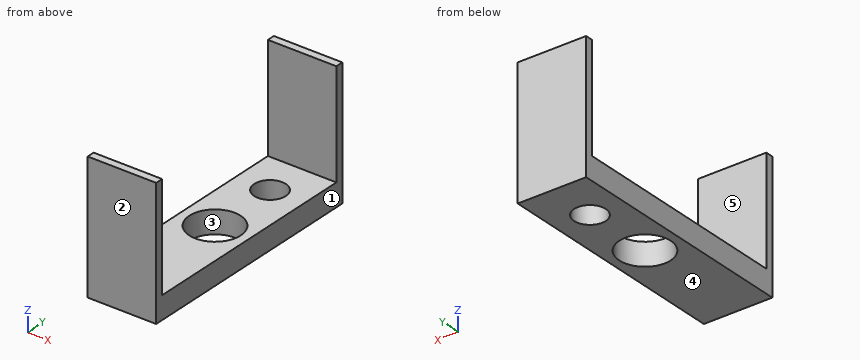
```python
from build123d import *

# Parameters (mm, degrees)
F0_W     = 24
F0_H     = 84.54
F1_DEPTH = 8
F2_W     = 24
F2_H     = 2.7
F3_DEPTH = 37.2
F4_R     = 9
F5_DEPTH = 8.001
F6_R     = 5.524405
F7_DEPTH = 8.001


with BuildPart() as f1:
    # F0 (on Top) → F1 (new body)
    with BuildSketch(Plane.XY):
        Rectangle(F0_W, F0_H)
    extrude(amount=F1_DEPTH)

    # F2 (on face) → F3 (join)
    with BuildSketch(Plane.XY.offset(8)):
        with Locations((0, 40.92)):
            Rectangle(F2_W, F2_H)
        with Locations((0, -40.92)):
            Rectangle(F2_W, F2_H)
    extrude(amount=F3_DEPTH)

    # F4 (on face) → F5 (cut, through all)
    with BuildSketch(Plane.XY.offset(8)):
        Circle(F4_R)
    extrude(amount=-F5_DEPTH, mode=Mode.SUBTRACT)

    # F6 (on face) → F7 (cut, through all)
    with BuildSketch(Plane.XY.offset(8)):
        with Locations((0, 25)):
            Circle(F6_R)
    extrude(amount=-F7_DEPTH, mode=Mode.SUBTRACT)


solid = f1.part
```
Can you work these out from the model? Positions are in its coordinate system, mm. Face numbers are marked on the shaded views. A direction names the side the tool comes from. Coordinates: 2 decimals unless noted, no trailing zeros. Order: outer loops, then holes, each group sorted by start corner. A loop starts at its lowest first (then second) coordinate and runs counter-clockwise, first axis right, second up.
1. If we section it at D-D (x = 7): Please give me the cut outline in (y, z), then the cut area to 3 significant figures.
2. Thinking about a two-plate mould opening in X: for the marked faces 1, 2 and 3, which applies, +X half, -X half, draft (parallel to the pull), parting line (faces both ways), or undercut?
3. If we section it at B-B (x = 0): Please give me the cut outline in (y, z), then the cut area to 3 significant figures.
4. For the marked faces 4 and 5, which set-ups out of +Z, -Z, +X, -X, +Y, -Y let a thin tool reach every point of the face, with its end or its side?
5. I need wall thicknesses on line 1 (Y direction, x = 0, z = 6.5); line 2 (Y direction, x = -6, z = 23); line 3 (Z direction, x = 1.75, y = -34). Which ranges of each line are inside material? Lowest first, please.
6. I'm going to push a flat-ended pin straight in: pin 1 (12 mm diameter, centred on x = 6, y = 7.5, fed in from +Z). Where does the tip first touch, or does it pass through?
7. If we section it at A-A (y = 0): Please give me the cut outline in (x, z), then the cut area to 3 significant figures.
8. If we section it at C-C (z = 9): Please give me the cut outline in (x, y).
Entries:
1. outline: (-42.27, 0) - (-5.66, 0) - (-5.66, 8) - (-39.57, 8) - (-39.57, 45.2) - (-42.27, 45.2) - close; (5.66, 0) - (42.27, 0) - (42.27, 45.2) - (39.57, 45.2) - (39.57, 8) - (5.66, 8) - close
1. area: 787 mm2
2. face 1: +X half
2. face 2: draft
2. face 3: undercut
3. outline: (-42.27, 0) - (-9, 0) - (-9, 8) - (-39.57, 8) - (-39.57, 45.2) - (-42.27, 45.2) - close; (9, 0) - (19.48, 0) - (19.48, 8) - (9, 8) - close; (30.52, 0) - (42.27, 0) - (42.27, 45.2) - (39.57, 45.2) - (39.57, 8) - (30.52, 8) - close
3. area: 645 mm2
4. face 4: -Z, +X, -X, +Y, -Y
4. face 5: +Z, +X, -X
5. line 1: y = -42.27 to -9, 9 to 19.48, 30.52 to 42.27
5. line 2: y = -42.27 to -39.57, 39.57 to 42.27
5. line 3: z = 0 to 8
6. pin 1: stops at z = 8
7. outline: (-12, 0) - (-9, 0) - (-9, 8) - (-12, 8) - close; (9, 0) - (12, 0) - (12, 8) - (9, 8) - close
7. area: 48.0 mm2
8. outline: (-12, -42.27) - (12, -42.27) - (12, -39.57) - (-12, -39.57) - close; (-12, 39.57) - (12, 39.57) - (12, 42.27) - (-12, 42.27) - close
